Read the model definition and answer for the solid it produces. Units are mm, in the model's axes. Face numbers are marked on the shaded views. A direction names the side the tool comes from. Coordinates: 2 decimals unless noted, no trailing zeros. Loops run counter-clockwise (first coordinate to the right, second up) from the corner with the lowest first, then second, coordinate; pieces in that order, holes last.
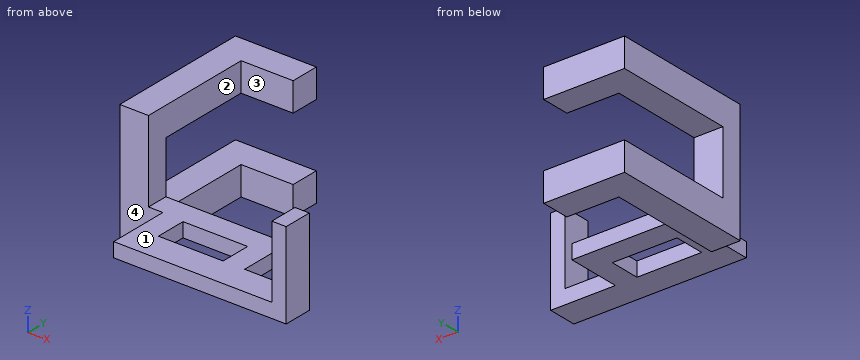
from build123d import *

# Parameters (mm, degrees)
SKETCH2_W                       = 38.1
SKETCH2_H                       = 29.21
BOSS_EXTRUDE1_DEPTH             = 5.08
SKETCH3_W                       = 22.86
SKETCH3_H                       = 12.7
CUT_EXTRUDE1_DEPTH              = 5.08
SKETCH5_W                       = 5.08
SKETCH5_H                       = 7.62
BOSS_EXTRUDE2_DEPTH             = 10.16
SKETCH7_W                       = 5.08
SKETCH7_H                       = 7.62
BOSS_EXTRUDE3_DEPTH             = 18.49
SKETCH8_W                       = 10.16
SKETCH8_H                       = 10.16
BOSS_EXTRUDE4_DEPTH             = 50.8
SKETCH9_W                       = 10.16
SKETCH9_H                       = 10.16
BOSS_EXTRUDE5_DEPTH             = 18.408905777
SKETCH11_W                      = 5.08
SKETCH11_H                      = 10.16
BOSS_EXTRUDE6_DEPTH             = 22.86
BOSS_EXTRUDE6_DIRECTION_2_REACH = 87.569
SKETCH12_W                      = 5.08
SKETCH12_H                      = 10.16
BOSS_EXTRUDE7_DEPTH             = 25.4
SKETCH13_W                      = 22.352
SKETCH13_H                      = 7.62
BOSS_EXTRUDE8_DEPTH             = 5.08


with BuildPart() as part:
    # Sketch2 → Boss-Extrude1 (new body)
    with BuildSketch(Plane.XY):
        Rectangle(SKETCH2_W, SKETCH2_H)
    extrude(amount=BOSS_EXTRUDE1_DEPTH)

    # Sketch3 → Cut-Extrude1 (cut)
    with BuildSketch(Plane.XY.offset(5.08)):
        Rectangle(SKETCH3_W, SKETCH3_H)
    extrude(amount=-CUT_EXTRUDE1_DEPTH, mode=Mode.SUBTRACT)

    # Sketch5 → Boss-Extrude2 (add)
    with BuildSketch(Plane.ZY.offset(19.05)):
        with Locations((2.54, 10.795)):
            Rectangle(SKETCH5_W, SKETCH5_H)
    extrude(amount=BOSS_EXTRUDE2_DEPTH)

    # Sketch7 → Boss-Extrude3 (add)
    with BuildSketch(Plane.XY.offset(5.08)):
        with Locations((-26.67, 10.795)):
            Rectangle(SKETCH7_W, SKETCH7_H)
    extrude(amount=BOSS_EXTRUDE3_DEPTH)

    # Sketch8 → Boss-Extrude4 (add)
    with BuildSketch(Plane.XZ.offset(-6.985)):
        with Locations((-29.21, 28.65)):
            Rectangle(SKETCH8_W, SKETCH8_H)
        with Locations((-29.21, -3.862)):
            Rectangle(SKETCH8_W, SKETCH8_H)
    extrude(amount=-BOSS_EXTRUDE4_DEPTH)

    # Sketch9 → Boss-Extrude5 (add)
    with BuildSketch(Plane(origin=(-24.13, 0, 0), x_dir=(0, 0, -1), z_dir=(1, 0, 0))):
        with Locations((-28.65, 52.705)):
            Rectangle(SKETCH9_W, SKETCH9_H)
        with Locations((3.862, 52.705)):
            Rectangle(SKETCH9_W, SKETCH9_H)
    extrude(amount=BOSS_EXTRUDE5_DEPTH)

    # Sketch11 → Boss-Extrude6 (add)
    with BuildSketch(Plane(origin=(19.05, 0, 0), x_dir=(0, 0, -1), z_dir=(1, 0, 0))):
        with Locations((-2.54, -9.525)):
            Rectangle(SKETCH11_W, SKETCH11_H)
    extrude(amount=BOSS_EXTRUDE6_DEPTH)

    # Sketch11 → Boss-Extrude6 direction 2 (add, up to next)
    with BuildSketch(Plane(origin=(19.05, 0, 0), x_dir=(0, 0, -1), z_dir=(1, 0, 0)), mode=Mode.PRIVATE) as boss_extrude6_direction_2_sk1:
        with Locations((-2.54, -9.525)):
            Rectangle(SKETCH11_W, SKETCH11_H)
    boss_extrude6_direction_2_tool1 = extrude(boss_extrude6_direction_2_sk1.sketch, amount=-BOSS_EXTRUDE6_DIRECTION_2_REACH, mode=Mode.PRIVATE) - part.part
    add(boss_extrude6_direction_2_tool1.solids().sort_by_distance((19.05, -9.525, 2.54))[0])

    # Sketch12 → Boss-Extrude7 (add)
    with BuildSketch(Plane.XY.offset(5.08)):
        with Locations((39.37, -9.525)):
            Rectangle(SKETCH12_W, SKETCH12_H)
    extrude(amount=BOSS_EXTRUDE7_DEPTH)

    # Sketch13 → Boss-Extrude8 (add)
    with BuildSketch(Plane.ZY.offset(29.21)):
        with Locations((12.394, 10.795)):
            Rectangle(SKETCH13_W, SKETCH13_H)
    extrude(amount=BOSS_EXTRUDE8_DEPTH)


solid = part.part
Q1. Flat-ended cylindrical pins translate along their axes: pin 1 Ø25 at (x, z) = (30.5, 14.5) entering from +Y (3 decimals); pin 2 Ø5.5 at (x, y) = (39, -8) entering from +Z; pin 3 Ø10 at (y, z) = (42.5, 15) entering from +X; pin 4 Ø9 at (x, y) = (11, 3) entering from -Z. Find the tip coordinate at first contact, or state that the pin passes through.
Findings below:
pin 1: stops at y = -4.445
pin 2: stops at z = 30.48
pin 3: passes through
pin 4: stops at z = 0
Q2. A cutting plane is placed at C-C (x = 6). Give the vertices of the cut face in (y, z) (3 decimals), then the cut area to 3 significant figures.
Findings below:
outline: (-14.605, 0) - (-4.445, 0) - (-4.445, 5.08) - (-14.605, 5.08) - close; (6.35, 0) - (14.605, 0) - (14.605, 5.08) - (6.35, 5.08) - close
area: 93.5 mm2
Q3. A cutting plane is placed at B-B (y = 45). Give the vertices of the cut face in (x, z), then the cut area to 3 significant figures.
Findings below:
outline: (-34.29, -8.94) - (-24.13, -8.94) - (-24.13, 1.22) - (-34.29, 1.22) - close; (-34.29, 23.57) - (-24.13, 23.57) - (-24.13, 33.73) - (-34.29, 33.73) - close
area: 206 mm2
Q4. A cutting plane is placed at D-D (x = -12.5). Give the vertices of the cut face in (y, z) (3 decimals), then the cut area to 3 significant figures.
Findings below:
outline: (-14.605, 0) - (14.605, 0) - (14.605, 5.08) - (-14.605, 5.08) - close; (47.625, -8.942) - (57.785, -8.942) - (57.785, 1.218) - (47.625, 1.218) - close; (47.625, 23.57) - (57.785, 23.57) - (57.785, 33.73) - (47.625, 33.73) - close
area: 355 mm2
Q5. Straight lines are drawn through the part: probe 1 along X at (y, z) = (-2, 5); probe 2 along Y at (x, z) = (-19, -5) (3 decimals); probe 3 along X at (y, z) = (39, -2). For each, find the intervals that lie inside material, in ascending order.
Findings below:
probe 1: x = -19.05 to -11.43, 11.43 to 19.05
probe 2: y = 47.625 to 57.785
probe 3: x = -34.29 to -24.13
Q6. A cutting plane is placed at A-A (z = 25.5). Give the vertices of the cut face in (x, y) (3 decimals).
Findings below:
outline: (-34.29, 6.985) - (-24.13, 6.985) - (-24.13, 47.625) - (-5.721, 47.625) - (-5.721, 57.785) - (-34.29, 57.785) - close; (36.83, -14.605) - (41.91, -14.605) - (41.91, -4.445) - (36.83, -4.445) - close
Q7. Which of the six approach directions +Z, -Z, +X, -X, +Y, -Y give full straight-line access (tool end or side, diameter ignored) to the marked faces 1, 2, 3 and 4?
Findings below:
face 1: +Z, +Y, -Y
face 2: +Z, +X, -Y
face 3: +Z, -Z, +X, -Y
face 4: +Z, -Z, -X, -Y
